Job drawing, mm, ordinate dimensions from the low corner. One solid piece. Round coordinates to 2 decimals unless told otherwise and drop trailing zeros. Write each loop counter-clockwise with the first axis right and the second up, starting at its lowest first coordinate (ties: lowest second). Pieces come first, ordered by that corner, then holes. Notation, with made-up numbers: (-5.75, 51) -> (9.25, 51) arc R7 cw to (9.25, 58) -> close; hole circle Ø4 at (75, 43). An arc over 180 degrees is marked (long way). Use CSV: the item, a comma, the result in double quotes. Start each with the question number.
(1) Saw through at B-B (z = 0.85). Give the cut face in (x, y), plus the area to 3 significant figures.
(2) Drop flat-ended pins along their axis: pin 1 (2 mm diameter, centred on x = 82.5, z = 3, fed in from -Y); pin 2 (1.5 mm diameter, centred on x = 98.5, z = 2, fed in from +Y); pin 3 (1 mm diameter, centred on x = 80, z = 0.5, fed in from +Y). Give the stop position or say it passes through.
(3) Saw through at C-C (y = 16). Give the cut face in (x, z).
(4) Probe line 1 (Y direction, x = 59, z = 2.35); line 2 (X direction, y = 2.25, z = 4.2); line 3 (Z direction, x = 51, y = 17.75). List the from-to ranges inside material, lowest first. Write a range as [from, to].
(5) Saw through at D-D (y = 3.5). Give the cut face in (x, z), plus the area to 3 significant figures.
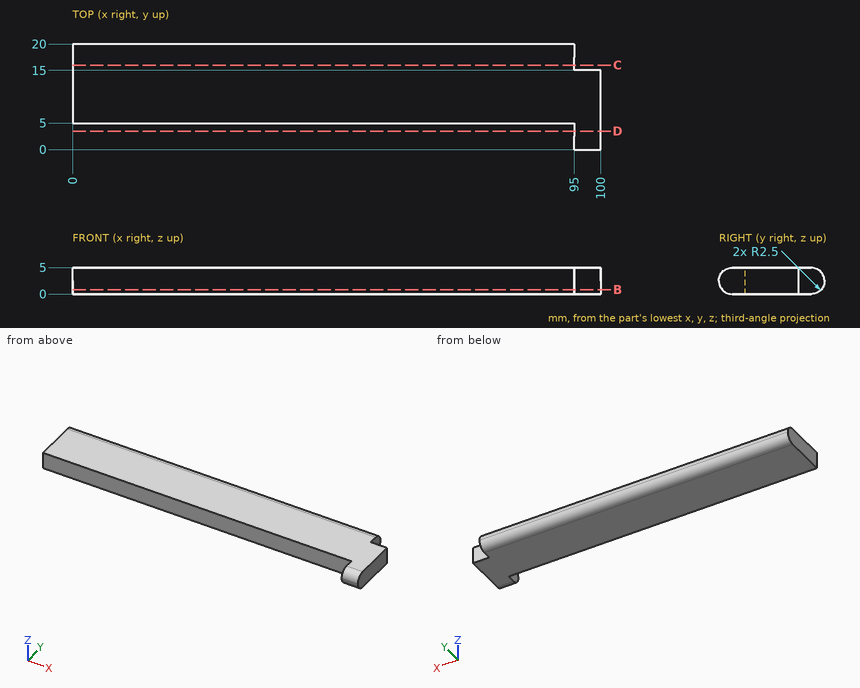
Answers:
1,outline,"(0, 5) -> (95, 5) -> (95, 0.62) -> (100, 0.62) -> (100, 15) -> (95, 15) -> (95, 19.38) -> (0, 19.38) -> close"
1,area,"1,440 mm²"
2,pin 1,"stops at y = 5"
2,pin 2,"stops at y = 15"
2,pin 3,"stops at y = 19.5"
3,outline,"(0, 0) -> (95, 0) -> (95, 5) -> (0, 5) -> close"
4,line 1,"y = [5, 20]"
4,line 2,"x = [95, 100]"
4,line 3,"z = [0.01, 4.99]"
5,outline,"(95, 0) -> (100, 0) -> (100, 5) -> (95, 5) -> close"
5,area,"25.0 mm²"
